Model file for the job. Use its own axes, mm. Coordinates: 2 decimals unless noted, no trailing zeros. Write each loop counter-clockwise with the first axis right and the second up, starting at its lowest first coordinate (ties: lowest second). Pieces come first, ordered by that corner, then holes. Notation, with made-up numbers: (-24.5, -32) -> (15.5, -32) arc R18 ccw to (15.5, -9) -> close; hole circle Ø8 at (60.25, 12). An arc over 180 degrees is marked (long way). Answer as a JSON object with one key per item and string values. Group by question number.
from build123d import *

# Parameters (mm, degrees)
SKETCH1_W                      = 75
SKETCH1_H                      = 12.7
BOSS_EXTRUDE1_DEPTH            = 12.7
M4_CLEARANCE_HOLE1_D           = 4.8
M4_CLEARANCE_HOLE1_CSINK_D     = 4.85
M4_CLEARANCE_HOLE1_CSINK_ANGLE = 100
M8_CLEARANCE_HOLE1_D           = 10
M8_CLEARANCE_HOLE1_CSINK_D     = 10.05
M8_CLEARANCE_HOLE1_CSINK_ANGLE = 100


with BuildPart() as part:
    # Sketch1 → Boss-Extrude1 (new body)
    with BuildSketch(Plane(origin=(0, 0, 0), x_dir=(1, 0, 0), z_dir=(0, 1, 0))):
        Rectangle(SKETCH1_W, SKETCH1_H)
    extrude(amount=BOSS_EXTRUDE1_DEPTH)

    # M4 Clearance Hole1 (through all)
    with Locations(Plane(origin=(0, 12.7, 0), x_dir=(1, 0, 0), z_dir=(0, 1, 0))):
        with Locations((-32, 0), (-22, 0), (22, 0), (32, 0)):
            CounterSinkHole(M4_CLEARANCE_HOLE1_D / 2, M4_CLEARANCE_HOLE1_CSINK_D / 2, counter_sink_angle=M4_CLEARANCE_HOLE1_CSINK_ANGLE)

    # M8 Clearance Hole1 (through all)
    with Locations(Plane.XY.offset(6.35)):
        with Locations((-3.5, 6.35), (3.5, 6.35)):
            CounterSinkHole(M8_CLEARANCE_HOLE1_D / 2, M8_CLEARANCE_HOLE1_CSINK_D / 2, counter_sink_angle=M8_CLEARANCE_HOLE1_CSINK_ANGLE)


solid = part.part
(1) Pull direction Y, two halves, no side cores. Call faces 1 (the face through (-1, 0, 0)), 2 (the face through (-34.217, 6.251, 0.919)), 3 (the face through (-8.497, 6.186, -0.099)): released by +Y, released by -Y, zero draft, split by the parting line, or undercut.
(2) Cut at D-D on x = -3.5. List the corners of the cut face in (y, z) (3 decimals), plus the area to 3 significant figures.
(3) Cut at B-B on x = 22. List the corners of the cut face in (y, z) (3 decimals).
(4) Wall check: probe 1 along X at (y, z) = (6.25, 5); probe 2 along X at (y, z) = (9, 1.5); probe 3 along X at (y, z) = (6.35, 1.75). Give the ranges that are in metal, low to high.
(5) Pin check, flat tip, straight feed: pin 1 (3 mm diameter, centred on x = 32, z = 0, fed in from -Y). Stop position of the tip, or through.
(6) Cut at A-A on y = 6.35. List the corners of the cut face in (x, z) (3 decimals).
(7) Cut at C-C on z = 0. Give the number of separate pieces and of enclosed holes in the cut face, plus the area to 3 significant figures.
Results found:
{
 "1": {"face 1": "released by -Y", "face 2": "zero draft", "face 3": "undercut"},
 "2": {"outline": "(0, -6.35) -> (1.35, -6.35) -> (1.35, 6.329) -> (1.325, 6.35) -> (0, 6.35) -> close; (11.35, -6.35) -> (12.7, -6.35) -> (12.7, 6.35) -> (11.375, 6.35) -> (11.35, 6.329) -> close", "area": "34.3 mm²"},
 "3": {"outline": "(0, -6.35) -> (12.7, -6.35) -> (12.7, -2.425) -> (12.679, -2.4) -> (0, -2.4) -> close; (0, 2.4) -> (12.679, 2.4) -> (12.7, 2.425) -> (12.7, 6.35) -> (0, 6.35) -> close"},
 "4": {"probe 1": "x = -37.5 to -8.5, 8.5 to 37.5", "probe 2": "x = -37.5 to -33.87, -30.13 to -23.87, -20.13 to -7.74, 7.74 to 20.13, 23.87 to 30.13, 33.87 to 37.5", "probe 3": "x = -37.5 to -33.64, -30.36 to -23.64, -20.36 to -8.5, 8.5 to 20.36, 23.64 to 30.36, 33.64 to 37.5"},
 "5": {"pin 1": "passes through"},
 "6": {"outline": "(-37.5, -6.35) -> (-8.5, -6.35) -> (-8.5, 6.329) -> (-8.525, 6.35) -> (-37.5, 6.35) -> close; (8.5, -6.35) -> (37.5, -6.35) -> (37.5, 6.35) -> (8.525, 6.35) -> (8.5, 6.329) -> close; hole circle Ø4.8 at (-32, 0); hole circle Ø4.8 at (-22, 0); hole circle Ø4.8 at (22, 0); hole circle Ø4.8 at (32, 0)"},
 "7": {"separate pieces": "5", "enclosed holes": "1", "area": "566 mm²"}
}
